from build123d import *

# Parameters (mm, degrees)
PAD_DEPTH    = 18
SKETCH001_W  = 18
SKETCH001_H  = 60
POCKET_DEPTH = 12
CHAMFER_SIZE = 15
FILLET_R     = 5
FILLET001_R  = 15
FILLET002_R  = 50


with BuildPart() as part:
    # Sketch → Pad (new body)
    with BuildSketch(Plane.XY):
        Polygon((0, 125), (0, -125), (96.630989, -111.4194), (115, -25), (115, 25), (96.630989, 111.4194), align=None)
    extrude(amount=PAD_DEPTH)

    # Sketch001 → Pocket (cut)
    with BuildSketch(Plane.XY.offset(18)):
        with Locations((55, 0)):
            Rectangle(SKETCH001_W, SKETCH001_H)
    extrude(amount=-POCKET_DEPTH, mode=Mode.SUBTRACT)

    # Chamfer
    chamfer_edges = [part.edges().sort_by_distance(p)[0] for p in [
        (0, -125, 9),
        (0, 125, 9),
    ]]
    chamfer(chamfer_edges, length=CHAMFER_SIZE)

    # Fillet
    fillet_edges = [part.edges().sort_by_distance(p)[0] for p in [
        (14.854021, 122.912403, 9),
        (0, 110, 9),
        (0, -110, 9),
        (14.854021, -122.912403, 9),
    ]]
    fillet(fillet_edges, radius=FILLET_R)

    # Fillet001
    fillet001_edges = [part.edges().sort_by_distance(p)[0] for p in [
        (96.630989, -111.4194, 9),
        (96.630989, 111.4194, 9),
    ]]
    fillet(fillet001_edges, radius=FILLET001_R)

    # Fillet002
    fillet002_edges = [part.edges().sort_by_distance(p)[0] for p in [
        (115, -25, 9),
        (115, 25, 9),
    ]]
    fillet(fillet002_edges, radius=FILLET002_R)


solid = part.part
Design review of the part built by this model. Coordinates are the model's own, in mm. A direction names the side the tool comes from. Round coordinates to 2 decimals unless told otherwise and drop trailing zeros. Loops run counter-clockwise (first coordinate to the right, second up) from the corner with the lowest first, then second, coordinate; pieces in that order, holes last. Notation, with made-up numbers: (79.25, -1) -> (131.25, -1) arc R3 ccw to (131.25, 4) -> close; hole circle Ø8 at (80.5, 64.25). An arc over 180 degrees is marked (long way). Use one line per item in the form item = value. Start each with the question number.
Q1. We need section A-A on z = 14.5. Give the boundary of the cut face in (x, y).
Q2. We need section B-B on z = 2.5. Give the boundary of the cut face in (x, y).
Q3. Wall thickness on line 1 along Z through (x, y) = (55, 11); line 2 along Y through (x, z) = (61.5, 16.75); line 3 along X through (y, z) = (29, 12): over which ranges is each line inside the solid? List them lowest first. Write a range as [from, to].
Q4. Machinability: for faces 1 (the face through (55, 0, 6)), 2 (the face through (44, 2, 18)), which of the approach directions +Z, -Z, +X, -X, +Y, -Y give a long, thin tool a straight path to every point of the face, cutting with its end or side? Answer none if there is none.
Q5. We need section C-C on x = 41.5. Give the boundary of the cut face in (y, z).
Q6. Draft analysis for pull direction Y (two halves, no side actions). For faces 3 (the face through (106.255, -66.14, 8.874)), 4 (the face through (64, 0, 12)), 5 (the face through (115, 0, 9)), state which applies: +Y half, -Y half, draft (parallel to the pull), parting line (faces both ways), or undercut.
Q7. We need section D-D on y = -39. Give the boundary of the cut face in (x, z).
Q8. For pin 1 Ø10 at (x, z) = (101.5, 12) entering from +Y; pin 2 Ø3 at (y, z) = (21.5, 4) entering from +X; pin 3 Ø9.5 at (x, z) = (58.5, 11) entering from -Y, all flat-tipped, find the tip position at first contact; note any pin that passes through.
Calculated:
q1.outline = (0, -107.72) arc R5 ccw to (1.72, -111.49) -> (13.13, -121.42) arc R5 ccw to (17.11, -122.6) -> (86.23, -112.88) arc R15 ccw to (98.81, -101.15) -> (113.91, -30.14) arc R50 ccw to (115, -19.74) -> (115, 19.74) arc R50 ccw to (113.91, 30.14) -> (98.81, 101.15) arc R15 ccw to (86.23, 112.88) -> (17.11, 122.6) arc R5 ccw to (13.13, 121.42) -> (1.72, 111.49) arc R5 ccw to (0, 107.72) -> close; hole (46, -30) -> (64, -30) -> (64, 30) -> (46, 30) -> close
q2.outline = (0, -107.72) arc R5 ccw to (1.72, -111.49) -> (13.13, -121.42) arc R5 ccw to (17.11, -122.6) -> (86.23, -112.88) arc R15 ccw to (98.81, -101.15) -> (113.91, -30.14) arc R50 ccw to (115, -19.74) -> (115, 19.74) arc R50 ccw to (113.91, 30.14) -> (98.81, 101.15) arc R15 ccw to (86.23, 112.88) -> (17.11, 122.6) arc R5 ccw to (13.13, 121.42) -> (1.72, 111.49) arc R5 ccw to (0, 107.72) -> close
q3.line_1 = [0, 6]
q3.line_2 = [-116.36, -30], [30, 116.36]
q3.line_3 = [0, 46], [64, 114.14]
q4.face_1 = +Z
q4.face_2 = +Z, +X, -X, +Y, -Y
q5.outline = (-119.17, 0) -> (119.17, 0) -> (119.17, 18) -> (-119.17, 18) -> close
q6.face_3 = -Y half
q6.face_4 = undercut
q6.face_5 = draft
q7.outline = (0, 0) -> (112.02, 0) -> (112.02, 18) -> (0, 18) -> close
q8.pin_1 = 106.53
q8.pin_2 = 115
q8.pin_3 = -117.45
